Can you work these out from the drawing? Everything is in mm from the part's minimum corner. Round coordinates to 2 decimals unless told otherwise and drop trailing zeros. Write each loop counter-clockwise with the first axis right and the second up, starting at its lowest first coordinate (ties: lowest second). Pieces come first, ordered by that corner, then holes. Notation, with made-up numbers: M 10,-24 L 52,-24 A12 ccw 52,-1 Z; hole C -5.75,-30.75 d10. An arc over 180 degrees is marked long. Use a Markdown table: item, result. Add a question column.
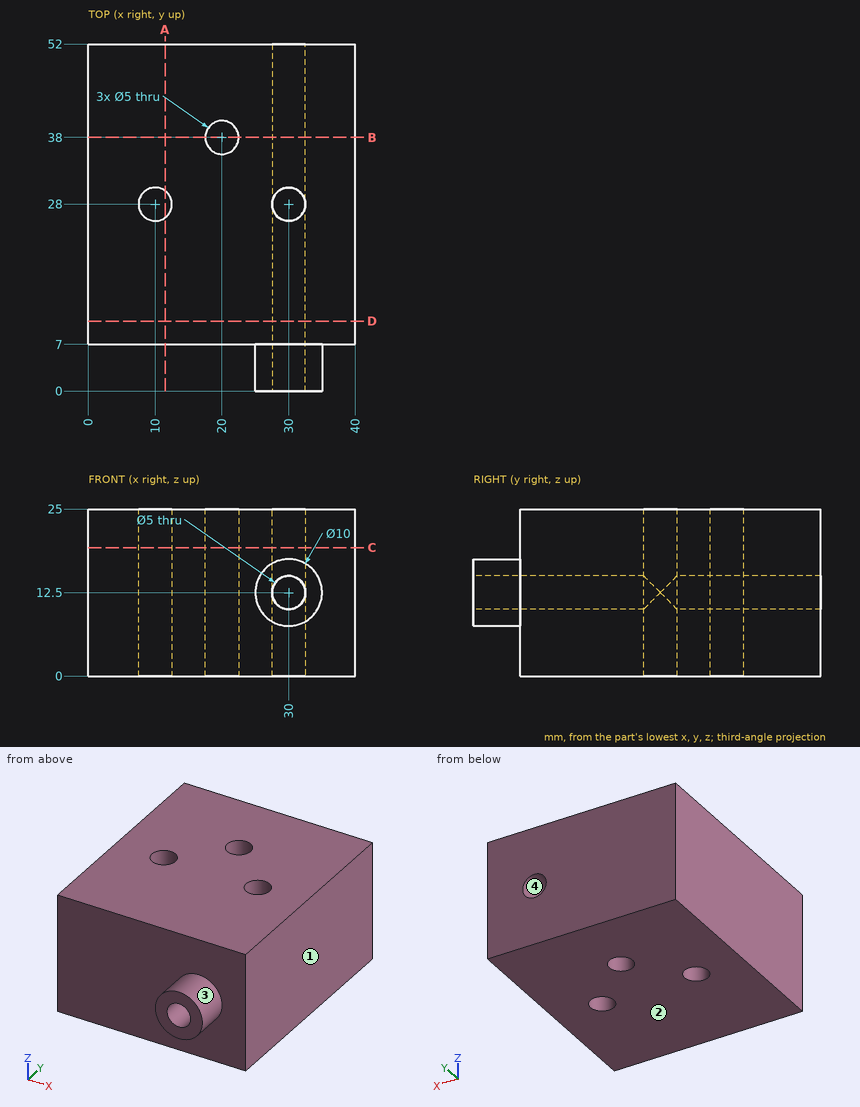
Item 1: I need wall thicknesses on probe 1 along Y at (x, z) = (20, 15); probe 2 along X at (y, z) = (36.5, 12.5); probe 3 along Z at (x, y) = (30, 33.25). Which ranges of each line are inside material? Lowest first, please. Write a range as from..to.
Item 2: If we mould it in two halves opening along Z, with no side actions, what happens to the marked faces 1, 2, 3 and 4? For each: +Z half, -Z half, draft (parallel to the pull), parting line (faces both ways), or undercut.
Item 3: Imagine slicing it at C-C on z = 19.25. List the corners of the cut face in (x, y) for me, plus the area to 3 significant figures.
Item 4: Imagine slicing it at A-A on x = 11.5. List the corners of the cut face in (y, z) for me.
Item 5: Imagine slicing it at B-B on y = 38. List the corners of the cut face in (x, z) for me, plus the area to 3 significant figures.
Item 6: Imagine slicing it at D-D on y = 10.5. List the corners of the cut face in (x, z) for me.
Item 7: For pin 1 Ø6 at (x, z) = (24, 2.5) entering from -Y, with a flat end and sliding along its axis, tell me the tip position at first contact or that it passes through.
The answers:
| question | item | result |
|---|---|---|
| 1 | probe 1 | 7..35.5, 40.5..52 |
| 1 | probe 2 | 0..18, 22..27.5, 32.5..40 |
| 1 | probe 3 | 0..10, 15..25 |
| 2 | face 1 | draft |
| 2 | face 2 | -Z half |
| 2 | face 3 | parting line |
| 2 | face 4 | undercut |
| 3 | outline | M 0,7 L 40,7 L 40,52 L 0,52 Z; hole C 10,28 d5; hole C 20,38 d5; hole C 30,28 d5 |
| 3 | area | 1,740 mm² |
| 4 | outline | M 7,0 L 26,0 L 26,25 L 7,25 Z; M 30,0 L 52,0 L 52,25 L 30,25 Z |
| 5 | outline | M 0,0 L 17.5,0 L 17.5,25 L 0,25 Z; M 22.5,0 L 40,0 L 40,25 L 22.5,25 Z; hole C 30,12.5 d5 |
| 5 | area | 855 mm² |
| 6 | outline | M 0,0 L 40,0 L 40,25 L 0,25 Z; hole C 30,12.5 d5 |
| 7 | pin 1 | y = 7 |
